Work out the finished part from the listing and answer in its coordinate system (mm). Face numbers are marked on the shaded views. Round coordinates to 2 decimals unless told otherwise and drop trailing zeros. Loops run counter-clockwise (first coordinate to the right, second up) from the corner with the lowest first, then second, coordinate; pieces in that order, holes last. Notation, with made-up numbers: (-36.75, 85) -> (20.25, 85) arc R22 ccw to (20.25, 103) -> close; hole circle Ø4 at (24, -6.75). An arc over 180 degrees is marked (long way). Use one line per item in the form item = value.
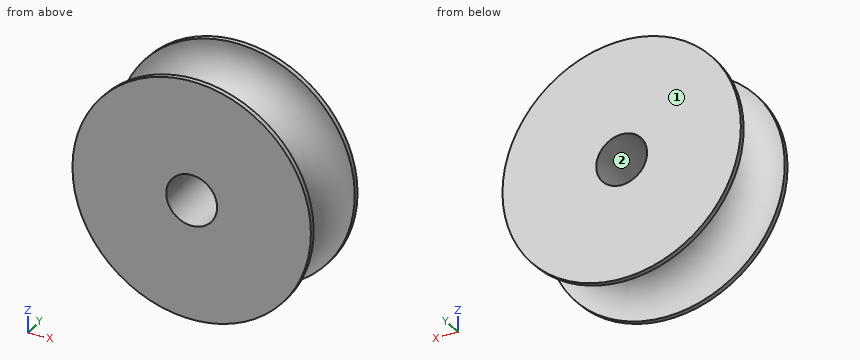
Autodesk Inventor part; units mm, degrees
ref_plane "YZ Plane" through (0, 0, 0) normal (1, 0, 0) x (0, 1, 0)
ref_plane "XZ Plane" through (0, 0, 0) normal (0, 1, 0) x (-1, 0, 0)
ref_plane "XY Plane" through (0, 0, 0) normal (0, 0, 1) x (1, 0, 0)
sketch "Sketch1" plane through (0, 0, 0) normal (0, 1, 0) x (-1, 0, 0)
  circle A0 centre (0, 0) radius 18.75
  dimension "d0" = 37.5
extrude "Extrusion1" add sketch "Sketch1" along normal blind 13
sketch "Sketch2" plane through (0, 0, 0) normal (1, 0, 0) x (0, 1, 0)
  line L0 (0, 0) -> (6.5, 0)
  line L1 (6.5, 0) -> (6.5, -11.875)
  circle A0 centre (6.5, -17.6902) radius 5.8152
  dimension "d3" = 6.5
  dimension "d4" = 11.875
revolve "Revolution1" cut sketch "Sketch2" angle 360 about axis through (0, 0, 0) along (0, 1, 0)
sketch "Sketch3" plane through (0, 0, 0) normal (0, -1, 0) x (1, 0, 0)
  circle A0 centre (0, 0) radius 4
  dimension "d6" = 8
extrude "Extrusion2" cut sketch "Sketch3" against normal through all
properties part number "pulleybearing"
(1) Given P1, Ø5, axis at y = 8.5, z = -6, coming from the +X side; P2, Ø5, axis at x = 10, y = 11, coming from the +Z side; P3, Ø6, axis at x = 13.5, y = 6, coming from the -Z side, each flat-ended and moving along its own axis, determine where each tip first touches the part or whether it passes through.
Completed:
P1 = 12.84
P2 = 17.04
P3 = -5.66
(2) Find section C-C, the plane y = 7.5. Write down the section's boundary in (x, z), then the cut area to 3 significant figures.
Completed:
outline = circle Ø23.92 at (0, 0); hole circle Ø8 at (0, 0)
area = 399 mm2
(3) Find section A-A, the plane z = 0. Write down the section's boundary in (x, y), then the cut area to 3 significant figures.
Completed:
outline = (-18.75, 0) -> (-4, 0) -> (-4, 13) -> (-18.75, 13) -> (-18.75, 12.22) arc R5.82 cw (long way) to (-18.75, 0.78) -> close; (4, 0) -> (18.75, 0) -> (18.75, 0.78) arc R5.82 cw (long way) to (18.75, 12.22) -> (18.75, 13) -> (4, 13) -> close
area = 253 mm2
(4) Find section B-B, the plane x = 0. Write down the section's boundary in (y, z), then the cut area to 3 significant figures.
Completed:
outline = (0, -18.75) -> (0.78, -18.75) arc R5.82 cw (long way) to (12.22, -18.75) -> (13, -18.75) -> (13, -4) -> (0, -4) -> close; (0, 4) -> (13, 4) -> (13, 18.75) -> (12.22, 18.75) arc R5.82 cw (long way) to (0.78, 18.75) -> (0, 18.75) -> close
area = 253 mm2
(5) Consider L1, parallel to Y at x = 14.5, z = 6; L2, parallel to Y at x = 6, z = -11; L3, parallel to Z at x = 0, y = 2.5. Determine where each line is inside the solid, lowest interval first.
Completed:
L1 = 0 to 1.04, 11.96 to 13
L2 = 0 to 3.82, 9.18 to 13
L3 = -13.47 to -4, 4 to 13.47
(6) Find section D-D, the plane y = 5. Write down the section's boundary in (x, z), then the cut area to 3 significant figures.
Completed:
outline = circle Ø24.14 at (0, 0); hole circle Ø8 at (0, 0)
area = 408 mm2
(7) For a pull along X with two mould halves and no side action, classify the marked faces 1 and 2 as +X half, -X half, draft (parallel to the pull), parting line (faces both ways), or undercut.
Completed:
face_1 = draft
face_2 = undercut
